Verification items for the finished model (mm, model axes). A direction names the side the tool comes from. Round coordinates to 2 decimals unless told otherwise and drop trailing zeros. Loops run counter-clockwise (first coordinate to the right, second up) from the corner with the lowest first, then second, coordinate; pieces in that order, holes last.
from build123d import *

# Parameters (mm, degrees)
F1_DEPTH  = 8.2
F2_W      = 14.3
F2_H      = 15.8
F3_DEPTH  = 10
F4_R      = 10.7
F5_DEPTH  = 4
F7_DEPTH  = 1
F8_R      = 3
F9_D      = 3.3
F9_DEPTH  = 4
F9_TIP    = 0.9914200214
F10_R     = 9
F11_DEPTH = 1.5
F12_R     = 11
F12_R_2   = 9
F13_DEPTH = 17


with BuildPart() as f1:
    # F0 (on Front) → F1 (new body)
    with BuildSketch(Plane.XZ):
        with BuildLine():
            ThreePointArc((40.55, 16.8), (39.2319805153, 19.9819805153), (36.05, 21.3))
            Line((36.05, 21.3), (-36.05, 21.3))
            ThreePointArc((-36.05, 21.3), (-39.2319805153, 19.9819805153), (-40.55, 16.8))
            Line((-40.55, 16.8), (-40.55, -16.8))
            ThreePointArc((-40.55, -16.8), (-39.2319805153, -19.9819805153), (-36.05, -21.3))
            Line((-36.05, -21.3), (36.05, -21.3))
            ThreePointArc((36.05, -21.3), (39.2319805153, -19.9819805153), (40.55, -16.8))
            Line((40.55, -16.8), (40.55, 16.8))
        make_face()
    extrude(amount=F1_DEPTH)

    # F2 (on face) → F3 (join)
    with BuildSketch(Plane(origin=(0, 0, 0), x_dir=(-1, 0, 0), z_dir=(0, 1, 0))):
        with Locations((-18.3, 0.1)):
            Rectangle(F2_W, F2_H)
    extrude(amount=F3_DEPTH)

    # F4 (on face) → F5 (join)
    with BuildSketch(Plane.XZ.offset(8.2)):
        with Locations((26.25, 0)):
            Circle(F4_R)
    extrude(amount=F5_DEPTH)

    # F6 (on face) → F7 (cut)
    with BuildSketch(Plane.XZ.offset(8.2)):
        Polygon((-32.55, 0), (-32.55, -17), (13.45, -17), (13.45, 17), (-32.55, 17), align=None)
    extrude(amount=-F7_DEPTH, mode=Mode.SUBTRACT)

    # F8
    f8_edges = [f1.edges().sort_by_distance(p)[0] for p in [
        (-40.55, -8.2, 0),
        (-39.231981, -8.2, -19.981981),
        (40.55, -8.2, 0),
    ]]
    fillet(f8_edges, radius=F8_R)

    # F9
    with Locations(Plane(origin=(0, 0, 0), x_dir=(1, 0, 0), z_dir=(0, 1, 0))):
        with Locations((37.2, -14.05), (36.05, 16.8), (-37.2, 14.05), (-37.2, -14.05)):
            Hole(F9_D / 2, depth=F9_DEPTH)
            with Locations((0, 0, -(F9_DEPTH + F9_TIP / 2))):  # 118° drill point
                Cone(0, F9_D / 2, F9_TIP, mode=Mode.SUBTRACT)

    # F10 (on face) → F11 (join)
    with BuildSketch(Plane.XZ.offset(12.2)):
        with Locations((26.25, 0)):
            Circle(F10_R)
    extrude(amount=F11_DEPTH)

    # F12 (on face) → F13 (join)
    with BuildSketch(Plane.XZ.offset(13.7)):
        with Locations((26.25, 0)):
            Circle(F12_R)
        with Locations((26.25, 0)):
            Circle(F12_R_2, mode=Mode.SUBTRACT)
        with Locations((26.25, 0)):
            Circle(F12_R_2)
    extrude(amount=F13_DEPTH)


solid = f1.part
1. Gauge pin test, flat ends, axial feed: P1, Ø6, axis at x = 27, z = -14, coming from the +Y side; P2, Ø12, axis at x = 27.5, y = -16, coming from the +Z side; P3, Ø2, axis at x = 37.2, z = 14.05, coming from the +Y side. Record the tip position at first contact, or that the pin passes through.
2. Scan lines: L1, parallel to X at y = -2.8, z = 14.05; L2, parallel to Z at x = -37.2, y = -2.35; L3, parallel to Z at x = 36.05, y = -1.95. Record each from-to range of solid material in increasing order.
3. Tool access check on faces 1 (the face through (18, 5, 8)), 2 (the face through (-35.89, -2.03, 15.05)), 3 (the face through (24, -12.2, 9)). Record the directions out of +Z, -Z, +X, -X, +Y, -Y that give a thin tool (end or side, any length) a straight path to the whole face; none if there is none.
4. Section check B-B (z = -6). Enter the section's corners in (x, y), then the cut area to 3 significant figures.
5. Section check A-A (x = 0). Enter the section's corners in (y, z), then the cut area to 3 significant figures.
6. Section check C-C (x = 26.5). Enter the section's corners in (y, z), then the cut area to 3 significant figures.
7. Release check for a two-part mould opening along Z. For faces 4 (the face through (26, -30.7, 0)), 5 (the face through (39.267, -2.564, 19.947)), 6 (the face through (-37.26, -4.82, 14.33)) record: released by +Z, released by -Z, zero draft, split by the parting line, or undercut.
Taken from the geometry:
1. P1: stops at y = 0
1. P2: stops at z = 11
1. P3: stops at y = -4.39
2. L1: x = -40.55 to -38.85, -35.55 to 35.55, 38.85 to 40.55
2. L2: z = -21.15 to -15.7, -12.4 to 12.4, 15.7 to 21.15
2. L3: z = -21.3 to -18.45, -15.15 to 12.87, 15.23 to 21.3
3. face 1: +Z, +X, -X, +Y
3. face 2: +Y
3. face 3: none
4. outline: (-40.55, -5.2) arc R3 ccw to (-37.55, -8.2) - (-32.55, -8.2) - (-32.55, -7.2) - (13.45, -7.2) - (13.45, -8.2) - (17.39, -8.2) - (17.39, -12.2) - (19.54, -12.2) - (19.54, -13.7) - (17.03, -13.7) - (17.03, -30.7) - (35.47, -30.7) - (35.47, -13.7) - (32.96, -13.7) - (32.96, -12.2) - (35.11, -12.2) - (35.11, -8.2) - (37.55, -8.2) arc R3 ccw to (40.55, -5.2) - (40.55, 0) - (25.45, 0) - (25.45, 10) - (11.15, 10) - (11.15, 0) - (-40.55, 0) - close
4. area: 1,160 mm2
5. outline: (-8.2, -18.3) arc R3 ccw to (-5.2, -21.3) - (0, -21.3) - (0, 21.3) - (-5.2, 21.3) arc R3 ccw to (-8.2, 18.3) - (-8.2, 17) - (-7.2, 17) - (-7.2, -17) - (-8.2, -17) - close
5. area: 311 mm2
6. outline: (-30.7, -11) - (-13.7, -11) - (-13.7, -9) - (-12.2, -9) - (-12.2, -10.7) - (-8.2, -10.7) - (-8.2, -18.3) arc R3 ccw to (-5.2, -21.3) - (0, -21.3) - (0, 21.3) - (-5.2, 21.3) arc R3 ccw to (-8.2, 18.3) - (-8.2, 10.7) - (-12.2, 10.7) - (-12.2, 9) - (-13.7, 9) - (-13.7, 11) - (-30.7, 11) - close
6. area: 832 mm2
7. face 4: zero draft
7. face 5: released by +Z
7. face 6: undercut
